from build123d import *

# Parameters (mm, degrees)
PAD001_DEPTH = 1.2
SKETCH007_W  = 16
SKETCH007_H  = 16
PAD002_DEPTH = 6.5
SKETCH008_R  = 1.5
PAD003_DEPTH = 15
SKETCH009_R  = 7
PAD004_DEPTH = 5
SKETCH010_W  = 18.8
SKETCH010_H  = 24
PAD005_DEPTH = 4.8


with BuildPart() as part:
    # Sketch006 → Pad001 (new body)
    with BuildSketch(Plane.XY):
        Polygon((-10.625, 72.5), (78.625, 72.5), (78.625, 65.575), (85, 65.575), (85, 20.925), (78.625, 20.925), (78.625, 14), (-10.625, 14), (-10.625, 20.925), (-17, 20.925), (-17, 65.575), (-10.625, 65.575), align=None)
    extrude(amount=PAD001_DEPTH)

    # Sketch007 (on Face14 of Pad001) → Pad002 (join)
    with BuildSketch(Plane.XY.offset(1.2)):
        with Locations((66.5, 62.9)):
            Rectangle(SKETCH007_W, SKETCH007_H)
    extrude(amount=PAD002_DEPTH)

    # Sketch008 (on Face5 of Pad002) → Pad003 (join)
    with BuildSketch(Plane.XY.offset(1.2)):
        with Locations((61.8, 39)):
            Circle(SKETCH008_R)
        with Locations((61.8, 35)):
            Circle(SKETCH008_R)
        with Locations((61.8, 31)):
            Circle(SKETCH008_R)
        with Locations((61.8, 27)):
            Circle(SKETCH008_R)
    extrude(amount=PAD003_DEPTH)

    # Sketch009 (on Face5 of Pad003) → Pad004 (join)
    with BuildSketch(Plane.XY.offset(1.2)):
        with Locations((73, 34)):
            Circle(SKETCH009_R)
    extrude(amount=PAD004_DEPTH)

    # Sketch010 (on Face5 of Pad004) → Pad005 (join)
    with BuildSketch(Plane.XY.offset(1.2)):
        with Locations((8.18, 58)):
            Rectangle(SKETCH010_W, SKETCH010_H)
    extrude(amount=PAD005_DEPTH)


with BuildPart() as part_1:
    # Body004 placement: moved
    add(part.part.moved(Location((0, 0, 4))))


solid = part_1.part
CAD build for the part. Positions are in the model's coordinates, mm. A direction names the side the tool comes from. Give positions to 0.01 mm unless a question says otherwise; leave off trailing zeros. Write each loop counter-clockwise with the first axis right and the second up, starting at its lowest first coordinate (ties: lowest second). Pieces come first, ordered by that corner, then holes. Notation, with made-up numbers: (-33.75, 30) - (13.25, 30) arc R15 cw to (13.25, 35) - close; hole circle Ø8 at (43, 29). An arc over 180 degrees is marked (long way). Put each result on its own line as item: value.
(1) Saw through at A-A (z = 7.5). List the corners of the cut face in (x, y), then the cut area to 3 significant figures.
Working result:
outline: (-1.22, 46) - (17.58, 46) - (17.58, 70) - (-1.22, 70) - close; (58.5, 54.9) - (74.5, 54.9) - (74.5, 70.9) - (58.5, 70.9) - close; circle Ø3 at (61.8, 27); circle Ø3 at (61.8, 31); circle Ø3 at (61.8, 35); circle Ø3 at (61.8, 39); circle Ø14 at (73, 34)
area: 889 mm^2
(2) Wall check: L1, parallel to X at y = 53, z = 5.75; L2, parallel to Z at x = 58, y = 27; L3, parallel to X at y = 26.5, z = 17. Give the ranges that are in metal, low to high.
Working result:
L1: -1.22 to 17.58
L2: 4 to 5.2
L3: 60.39 to 63.21
(3) Saw through at D-D (z = 13). List the corners of the cut face in (x, y), then the cut area to 3 significant figures.
Working result:
outline: circle Ø3 at (61.8, 27); circle Ø3 at (61.8, 31); circle Ø3 at (61.8, 35); circle Ø3 at (61.8, 39)
area: 28.3 mm^2
(4) Saw through at B-B (y = 69). List the corners of the cut face in (x, z) (3 decimals).
Working result:
outline: (-10.625, 4) - (78.625, 4) - (78.625, 5.2) - (74.5, 5.2) - (74.5, 11.7) - (58.5, 11.7) - (58.5, 5.2) - (17.58, 5.2) - (17.58, 10) - (-1.22, 10) - (-1.22, 5.2) - (-10.625, 5.2) - close
(5) Tool access for faces 1 (the cylindrical face through (67.84, 38.73, 7.66)), 2 (the flat face through (58.5, 63, 8)), 3 (the flat face through (8, 46, 8)): list every direction of +Z, -Z, +X, -X, +Y, -Y with a clear straight run to the whole face (end or side of a thin tool).
Working result:
face 1: +Z
face 2: +Z, +Y, -Y
face 3: +Z, +X, -X, -Y
(6) Drop flat-ended pins along their axis: pin 1 Ø3 at (y, z) = (65, 8) entering from -X; pin 2 Ø5 at (x, z) = (63, 9) entering from +Y; pin 3 Ø1.4 at (x, z) = (6.5, 7.5) entering from +Y. Give the stop position or say it passes through.
Working result:
pin 1: x = -1.22
pin 2: y = 70.9
pin 3: y = 70
(7) Saw through at C-C (x = 61.8). List the corners of the cut face in (y, z).
Working result:
outline: (14, 4) - (72.5, 4) - (72.5, 5.2) - (70.9, 5.2) - (70.9, 11.7) - (54.9, 11.7) - (54.9, 5.2) - (40.5, 5.2) - (40.5, 20.2) - (37.5, 20.2) - (37.5, 5.2) - (36.5, 5.2) - (36.5, 20.2) - (33.5, 20.2) - (33.5, 5.2) - (32.5, 5.2) - (32.5, 20.2) - (29.5, 20.2) - (29.5, 5.2) - (28.5, 5.2) - (28.5, 20.2) - (25.5, 20.2) - (25.5, 5.2) - (14, 5.2) - close
(8) Pull direction Y, two halves, no side cores. Call faces 4 (the flat face through (8, 58, 10)), 5 (the cylindrical face through (60.6, 30.1, 12.6)), 6 (the flat face through (8, 70, 8)): released by +Y, released by -Y, zero draft, split by the parting line, or undercut.
Working result:
face 4: zero draft
face 5: undercut
face 6: released by +Y
